Verification items for the finished model (mm, model axes). A direction names the side the tool comes from. Give positions to 0.01 mm unless a question says otherwise; leave off trailing zeros. Write each loop counter-clockwise with the first axis right and the second up, starting at its lowest first coordinate (ties: lowest second). Pieces come first, ordered by that corner, then holes. Notation, with made-up numbers: (-25.75, -10) -> (31.25, -10) arc R23 cw to (31.25, 6) -> close; hole circle Ø7 at (9.25, 16). An arc over 180 degrees is marked (long way). Use CSV: the item, a comma, the result in double quotes. Start each with the question number.
```python
from build123d import *

# Parameters (mm, degrees)
SKETCH2_W                = 360
SKETCH2_H                = 220
BOSS_EXTRUDE1_DEPTH      = 480
SKETCH4_W                = 280
SKETCH4_H                = 110
CUT_EXTRUDE2_DEPTH       = 470
SKETCH5_W                = 110
SKETCH5_H                = 460
CUT_EXTRUDE3_DEPTH       = 40
SKETCH6_W                = 340
SKETCH6_H                = 100
CUT_EXTRUDE4_DEPTH       = 50
SKETCH7_W                = 340
SKETCH7_H                = 10
CUT_EXTRUDE5_DEPTH       = 420
SKETCH8_W                = 340
SKETCH8_H                = 410
CUT_EXTRUDE6_DEPTH       = 90
SKETCH12_W               = 10
SKETCH12_H               = 20
CUT_EXTRUDE9_DEPTH       = 10
CUT_EXTRUDE11_DEPTH      = 470
CUT_EXTRUDE11_DEPTH_BACK = 10
SKETCH18_W               = 100
SKETCH18_H               = 50
SKETCH23_W               = 110
SKETCH23_H               = 460
CUT_EXTRUDE13_DEPTH      = 20
SKETCH24_W               = 20
SKETCH24_H               = 110
CUT_EXTRUDE14_DEPTH      = 10
SKETCH26_R               = 5
CUT_EXTRUDE15_DEPTH      = 480
CUT_EXTRUDE16_DEPTH      = 480
SKETCH28_W               = 340
SKETCH28_H               = 10
CUT_EXTRUDE17_DEPTH      = 100
CHAMFER1_SIZE            = 10
CHAMFER2_SIZE            = 10
FILLET2_R                = 10
CHAMFER3_SIZE            = 10
FILLET4_R                = 2
FILLET5_R                = 2
CHAMFER4_SIZE            = 10
SKETCH29_W               = 340
SKETCH29_H               = 24.70137943
CUT_EXTRUDE18_DEPTH      = 10
SKETCH30_W               = 300
SKETCH30_H               = 27.571183361
CUT_EXTRUDE19_DEPTH      = 10


# Some blends are built 0.0001 mm under size
with BuildPart() as part:
    # Sketch2 → Boss-Extrude1 (new body)
    with BuildSketch(Plane(origin=(0, 0, 0), x_dir=(1, 0, 0), z_dir=(0, 1, 0))):
        with Locations((-139.181984943, -115.021725484)):
            Rectangle(SKETCH2_W, SKETCH2_H)
    extrude(amount=BOSS_EXTRUDE1_DEPTH)

    # Sketch4 → Cut-Extrude2 (cut)
    with BuildSketch(Plane(origin=(0, 480, 0), x_dir=(1, 0, 0), z_dir=(0, 1, 0))):
        with Locations((-129.181984943, -170.021725484)):
            Rectangle(SKETCH4_W, SKETCH4_H)
    extrude(amount=-CUT_EXTRUDE2_DEPTH, mode=Mode.SUBTRACT)

    # Sketch5 → Cut-Extrude3 (cut)
    with BuildSketch(Plane(origin=(-269.181984943, 0, 0), x_dir=(0, 0, -1), z_dir=(1, 0, 0))):
        with Locations((-170.021725484, 240)):
            Rectangle(SKETCH5_W, SKETCH5_H)
    extrude(amount=-CUT_EXTRUDE3_DEPTH, mode=Mode.SUBTRACT)

    # Sketch6 → Cut-Extrude4 (cut)
    with BuildSketch(Plane(origin=(0, 480, 0), x_dir=(1, 0, 0), z_dir=(0, 1, 0))):
        with Locations((-139.181984943, -55.021725484)):
            Rectangle(SKETCH6_W, SKETCH6_H)
    extrude(amount=-CUT_EXTRUDE4_DEPTH, mode=Mode.SUBTRACT)

    # Sketch7 → Cut-Extrude5 (cut)
    with BuildSketch(Plane(origin=(0, 430, 0), x_dir=(1, 0, 0), z_dir=(0, 1, 0))):
        with Locations((-139.181984943, -100.021725484)):
            Rectangle(SKETCH7_W, SKETCH7_H)
    extrude(amount=-CUT_EXTRUDE5_DEPTH, mode=Mode.SUBTRACT)

    # Sketch8 → Cut-Extrude6 (cut)
    with BuildSketch(Plane(origin=(0, 0, 5.021725484), x_dir=(-1, 0, 0), z_dir=(0, 0, -1))):
        with Locations((139.181984943, 215)):
            Rectangle(SKETCH8_W, SKETCH8_H)
    extrude(amount=-CUT_EXTRUDE6_DEPTH, mode=Mode.SUBTRACT)

    # Sketch12 → Cut-Extrude9 (cut)
    with BuildSketch(Plane(origin=(0, 0, 105.021725484), x_dir=(-1, 0, 0), z_dir=(0, 0, -1))):
        with Locations((-25.818015057, 240)):
            Rectangle(SKETCH12_W, SKETCH12_H)
        with Locations((304.181984943, 240)):
            Rectangle(SKETCH12_W, SKETCH12_H)
    extrude(amount=-CUT_EXTRUDE9_DEPTH, mode=Mode.SUBTRACT)

    # Sketch18 → Cut-Extrude11 (cut, two sides: drawn at the far end of the back side and taken through both)
    with BuildSketch(Plane(origin=(-309.181984943, 0, 0), x_dir=(0, 0, -1), z_dir=(1, 0, 0)).offset(-CUT_EXTRUDE11_DEPTH_BACK)):
        with Locations((-55.021725484, 455)):
            Rectangle(SKETCH18_W, SKETCH18_H)
    extrude(amount=CUT_EXTRUDE11_DEPTH + CUT_EXTRUDE11_DEPTH_BACK, mode=Mode.SUBTRACT)

    # Sketch23 → Cut-Extrude13 (cut)
    with BuildSketch(Plane.ZY.offset(-10.818015057)):
        with Locations((170.021725484, 240)):
            Rectangle(SKETCH23_W, SKETCH23_H)
    extrude(amount=-CUT_EXTRUDE13_DEPTH, mode=Mode.SUBTRACT)

    # Sketch24 → Cut-Extrude14 (cut)
    with BuildSketch(Plane(origin=(0, 480, 0), x_dir=(1, 0, 0), z_dir=(0, 1, 0))):
        with Locations((-279.181984943, -170.021725484)):
            Rectangle(SKETCH24_W, SKETCH24_H)
    extrude(amount=-CUT_EXTRUDE14_DEPTH, mode=Mode.SUBTRACT)

    # Sketch26 → Cut-Extrude15 (cut)
    with BuildSketch(Plane(origin=(40.818015057, 0, 0), x_dir=(0, 0, -1), z_dir=(1, 0, 0))):
        with Locations((-205.021725484, 240)):
            Circle(SKETCH26_R)
    extrude(amount=-CUT_EXTRUDE15_DEPTH, mode=Mode.SUBTRACT)

    # Sketch27 → Cut-Extrude16 (cut)
    with BuildSketch(Plane(origin=(40.818015057, 0, 0), x_dir=(0, 0, -1), z_dir=(1, 0, 0))):
        Polygon((-15.021725484, 335), (-95.021725484, 415), (-15.021725484, 415), align=None)
        Polygon((-15.021725484, 322.5), (-95.021725484, 402.5), (-95.021725484, 322.5), align=None)
        Polygon((-15.021725484, 312.5), (-95.021725484, 232.5), (-95.021725484, 312.5), align=None)
        Polygon((-15.021725484, 220), (-15.021725484, 300), (-95.021725484, 220), align=None)
        Polygon((-15.021725484, 130), (-95.021725484, 210), (-15.021725484, 210), align=None)
        Polygon((-95.021725484, 117.5), (-95.021725484, 197.5), (-15.021725484, 117.5), align=None)
        Polygon((-15.021725484, 107.5), (-95.021725484, 27.5), (-95.021725484, 107.5), align=None)
        Polygon((-15.021725484, 15), (-15.021725484, 95), (-95.021725484, 15), align=None)
    extrude(amount=-CUT_EXTRUDE16_DEPTH, mode=Mode.SUBTRACT)

    # Sketch28 → Cut-Extrude17 (cut)
    with BuildSketch(Plane(origin=(0, 0, 5.021725484), x_dir=(-1, 0, 0), z_dir=(0, 0, -1))):
        with Locations((139.181984943, 5)):
            Rectangle(SKETCH28_W, SKETCH28_H)
    extrude(amount=-CUT_EXTRUDE17_DEPTH, mode=Mode.SUBTRACT)

    # Chamfer1
    chamfer1_edges = [part.edges().sort_by_distance(p)[0] for p in [
        (40.818015057, 430, 55.021725484),
        (-319.181984943, 430, 55.021725484),
    ]]
    chamfer(chamfer1_edges, length=CHAMFER1_SIZE - 0.0001)  # a hair under: the kernel refuses the full size

    # Chamfer2
    chamfer2_edges = [part.edges().sort_by_distance(p)[0] for p in [
        (-319.181984943, 480, 165.021725484),
        (40.818015057, 480, 165.021725484),
    ]]
    chamfer(chamfer2_edges, length=CHAMFER2_SIZE)

    # Fillet2
    fillet2_edges = [part.edges().sort_by_distance(p)[0] for p in [
        (-139.181984943, 480, 105.021725484),
    ]]
    fillet(fillet2_edges, radius=FILLET2_R - 0.0001)  # a hair under: the kernel refuses the full size

    # Chamfer3
    # the kernel refuses this chamfer: 10 mm, written as the material it takes off along each edge
    with BuildSketch(Plane(origin=(-319.181984943, 495.71682988, 105.021725484), x_dir=(0.9996219169112968, 0, -0.027495876610586282), z_dir=(0, -1, 0))) as chamfer3_piece_1_section:
        Polygon((CHAMFER3_SIZE * 0.999621916911, CHAMFER3_SIZE * 0.0274958766106), (-CHAMFER3_SIZE * 0.0274958766106, CHAMFER3_SIZE * 0.999621916911), (0, 0), align=None)
    chamfer3_piece_1 = extrude(amount=101.433559759, mode=Mode.PRIVATE)
    chamfer3_piece_1 = split(chamfer3_piece_1, bisect_by=Plane(origin=(-315.895641605, 430, 108.325767027), z_dir=(0, 1, 0)), keep=Keep.TOP, mode=Mode.PRIVATE)
    chamfer3_piece_1 = split(chamfer3_piece_1, bisect_by=Plane(origin=(-309.181984943, 462.85841494, 108.325767027), z_dir=(-1, 0, 0)), keep=Keep.TOP, mode=Mode.PRIVATE)
    add(chamfer3_piece_1, mode=Mode.SUBTRACT)
    with BuildSketch(Plane(origin=(-319.181984943, 495.71682988, 105.021725484), x_dir=(0.9996219169112968, 0, -0.027495876610586282), z_dir=(0, -1, 0))) as chamfer3_piece_2_section:
        Polygon((CHAMFER3_SIZE * 0.999621916911, CHAMFER3_SIZE * 0.0274958766106), (-CHAMFER3_SIZE * 0.0274958766106, CHAMFER3_SIZE * 0.999621916911), (0, 0), align=None)
    chamfer3_piece_2 = extrude(amount=101.433559759, mode=Mode.PRIVATE)
    chamfer3_piece_2 = split(chamfer3_piece_2, bisect_by=Plane(origin=(-314.919016281, 424.263068662, 108.826082354), z_dir=(-0.7071067811865476, 0.7071067811865476, 0)), keep=Keep.TOP, mode=Mode.PRIVATE)
    chamfer3_piece_2 = split(chamfer3_piece_2, bisect_by=Plane(origin=(-316.831326727, 430, 108.826082354), z_dir=(0, -1, 0)), keep=Keep.TOP, mode=Mode.PRIVATE)
    add(chamfer3_piece_2, mode=Mode.SUBTRACT)
    with BuildSketch(Plane(origin=(40.818015057, 394.28327012, 105.021725484), x_dir=(-0.9996219169112968, 0, -0.027495876610586317), z_dir=(0, 1, 0))) as chamfer3_piece_3_section:
        Polygon((CHAMFER3_SIZE * 0.999621916911, CHAMFER3_SIZE * 0.0274958766106), (-CHAMFER3_SIZE * 0.0274958766106, CHAMFER3_SIZE * 0.999621916911), (0, 0), align=None)
    chamfer3_piece_3 = extrude(amount=101.433559759, mode=Mode.PRIVATE)
    chamfer3_piece_3 = split(chamfer3_piece_3, bisect_by=Plane(origin=(36.555046395, 424.263068662, 108.826082354), z_dir=(0.7071067811865485, 0.7071067811865467, 0)), keep=Keep.TOP, mode=Mode.PRIVATE)
    chamfer3_piece_3 = split(chamfer3_piece_3, bisect_by=Plane(origin=(38.46735684, 430, 108.826082354), z_dir=(0, -1, 0)), keep=Keep.TOP, mode=Mode.PRIVATE)
    add(chamfer3_piece_3, mode=Mode.SUBTRACT)
    with BuildSketch(Plane(origin=(40.818015057, 394.28327012, 105.021725484), x_dir=(-0.9996219169112968, 0, -0.027495876610586317), z_dir=(0, 1, 0))) as chamfer3_piece_4_section:
        Polygon((CHAMFER3_SIZE * 0.999621916911, CHAMFER3_SIZE * 0.0274958766106), (-CHAMFER3_SIZE * 0.0274958766106, CHAMFER3_SIZE * 0.999621916911), (0, 0), align=None)
    chamfer3_piece_4 = extrude(amount=101.433559759, mode=Mode.PRIVATE)
    chamfer3_piece_4 = split(chamfer3_piece_4, bisect_by=Plane(origin=(37.531671719, 430, 108.325767027), z_dir=(0, 1, 0)), keep=Keep.TOP, mode=Mode.PRIVATE)
    chamfer3_piece_4 = split(chamfer3_piece_4, bisect_by=Plane(origin=(30.818015057, 462.85841494, 108.325767027), z_dir=(1, 0, 0)), keep=Keep.TOP, mode=Mode.PRIVATE)
    add(chamfer3_piece_4, mode=Mode.SUBTRACT)

    # Fillet4
    fillet4_edges = [part.edges().sort_by_distance(p)[0] for p in [
        (-139.181984943, 0, 105.021725484),
        (-309.181984943, 0, 55.021725484),
        (30.818015057, 0, 55.021725484),
        (-139.181984943, 430, 5.021725484),
        (30.818015057, 210, 5.021725484),
        (-139.181984943, 420, 5.021725484),
        (-309.181984943, 210, 5.021725484),
    ]]
    fillet(fillet4_edges, radius=FILLET4_R)

    # Fillet5
    fillet5_edges = [part.edges().sort_by_distance(p)[0] for p in [
        (-139.181984943, 430, 95.021725484),
    ]]
    fillet(fillet5_edges, radius=FILLET5_R)

    # Chamfer4
    # the kernel refuses this chamfer: 10 mm, written as the material it takes off along each edge
    with BuildSketch(Plane(origin=(-319.181984943, 0, 250.738555364), x_dir=(0.9996219169112968, -0.027495876610586334, 0), z_dir=(0, 0, -1))) as chamfer4_piece_1:
        Polygon((CHAMFER4_SIZE * 0.999621916911, -CHAMFER4_SIZE * 0.0274958766106), (-CHAMFER4_SIZE * 0.0274958766106, -CHAMFER4_SIZE * 0.999621916911), (0, 0), align=None)
    extrude(amount=271.433659759, mode=Mode.SUBTRACT)
    with BuildSketch(Plane(origin=(40.818015057, 0, -20.695104396), x_dir=(0.027495876610586317, 0.9996219169112968, 0), z_dir=(0, 0, 1))) as chamfer4_piece_2:
        Polygon((CHAMFER4_SIZE * 0.999621916911, CHAMFER4_SIZE * 0.0274958766106), (-CHAMFER4_SIZE * 0.0274958766106, CHAMFER4_SIZE * 0.999621916911), (0, 0), align=None)
    extrude(amount=271.433659759, mode=Mode.SUBTRACT)

    # Sketch29 → Cut-Extrude18 (cut)
    with BuildSketch(Plane(origin=(0, 0, 105.021725484), x_dir=(-1, 0, 0), z_dir=(0, 0, -1))):
        with Locations((139.181984943, 457.649310285)):
            Rectangle(SKETCH29_W, SKETCH29_H)
    extrude(amount=-CUT_EXTRUDE18_DEPTH, mode=Mode.SUBTRACT)

    # Sketch30 → Cut-Extrude19 (cut)
    with BuildSketch(Plane(origin=(0, 480, 0), x_dir=(1, 0, 0), z_dir=(0, 1, 0))):
        with Locations((-139.181984943, -101.236133803)):
            Rectangle(SKETCH30_W, SKETCH30_H)
    extrude(amount=-CUT_EXTRUDE19_DEPTH, mode=Mode.SUBTRACT)


solid = part.part
```
(1) Draft check along X on faces 1 (the face through (-140, 8, 225.022)), 2 (the face through (35.75, 425.07, 60.79)), 3 (the face through (26, 230, 110)). Enter one of: released by +X, released by -X, zero draft, split by the parting line, or undercut.
(2) Section check B-B on z = 170. Record the cut outline in (x, y), then the cut area to 3 significant figures.
(3) Section check C-C on y = 363. Give the number of separate pieces and of enclosed holes in the cut face, then the cut area to 3 significant figures.
(4) Thickness scan on line 1 (Z direction, x = -144, y = 427.5); line 2 (X direction, y = 48, z = 125); line 3 (Y direction, x = 6.5, z = 40.5). Record the ranges inside material, lowest first. Write a range as from..to.
(5) Set-up check for faces 4 (the face through (35.89, 5.07, 113.48)), 5 (the face through (20.818, 240, 110)), 6 (the face through (36, 220, 56)): record each of +Z, -Z, +X, -X, +Y, -Y from which the full face is reachable in a straight line by a thin tool's end or side.
(6) Go/stop test with flat-tipped pins: pin 1 (5 mm diameter, centred on x = -314, z = 53.5, fed in from -Y); pin 2 (5 mm diameter, centred on x = -314.5, z = 70, fed in from -Y); pin 3 (10 mm diameter, centred on x = -22, z = 72, fed in from -Y). Record where each tip stops, or that it passes through.
(7) Section check A-A on x = -80. Record the cut outline in (y, z), then the cut area to 3 significant figures.
Data:
1,face 1,"zero draft"
1,face 2,"released by +X"
1,face 3,"undercut"
2,outline,"(-319.18, 10) -> (-309.18, 0) -> (30.82, 0) -> (40.82, 10) -> (40.82, 470) -> (30.82, 480) -> (10.82, 480) -> (10.82, 470) -> (30.82, 470) -> (30.82, 10) -> (-309.18, 10) -> (-309.18, 470) -> (-289.18, 470) -> (-289.18, 480) -> (-309.18, 480) -> (-319.18, 470) -> close"
2,area,"13,200 mm2"
3,separate pieces,"5"
3,enclosed holes,"0"
3,area,"6,450 mm2"
4,line 1,"z = 5.02..95.02, 105.02..115.02"
4,line 2,"x = -319.18..-309.18, 30.82..40.82"
4,line 3,"y = 420..430"
5,face 4,"+Z, -Z, +X, -Y"
5,face 5,"+Z, -Z"
5,face 6,"+X, -X"
6,pin 1,"stops at y = 2.32"
6,pin 2,"stops at y = 2.82"
6,pin 3,"stops at y = 420"
7,outline,"(0, 107.02) arc R2 ccw to (2, 105.02) -> (445.3, 105.02) -> (445.3, 115.02) -> (10, 115.02) -> (10, 225.02) -> (0, 225.02) -> close; (420, 7.02) arc R2 ccw to (422, 5.02) -> (428, 5.02) arc R2 ccw to (430, 7.02) -> (430, 93.02) arc R2 ccw to (428, 95.02) -> (420, 95.02) -> close"
7,area,"6,450 mm2"
